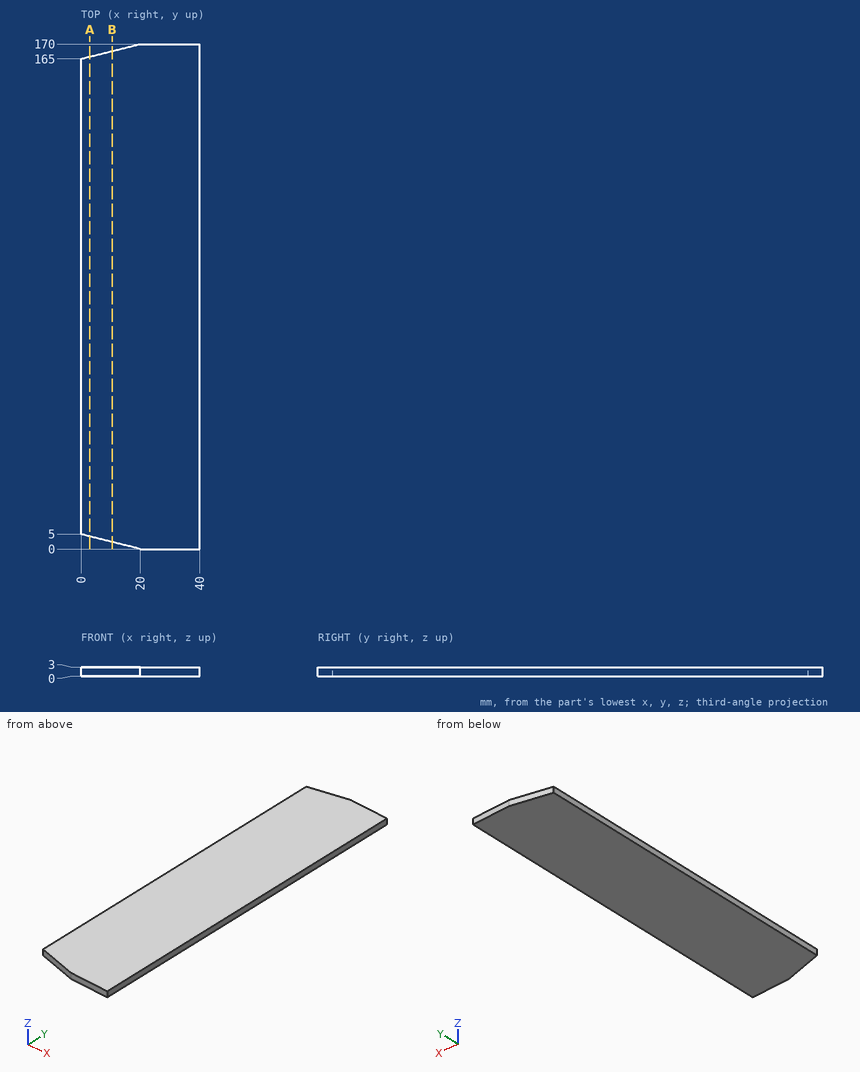
Geometry check sheet. Reference: drawing and pictorial views, mm from the part's lowest x, y, z. Round coordinates to 2 decimals unless told otherwise and drop trailing zeros. Loops run counter-clockwise (first coordinate to the right, second up) from the corner with the lowest first, then second, coordinate; pieces in that order, holes last. Notation, with made-up numbers: (62.25, -32.75) - (111.25, -32.75) arc R24 ccw to (111.25, -6.75) - close; hole circle Ø6 at (64.25, -37). An arc over 180 degrees is marked (long way). Answer in a Markdown table with one row per item. Add a question column.
Q1. Section check B-B on x = 10.5. Enter the section's corners in (y, z) (3 decimals), plus the area to 3 significant figures.
Q2. Material ranges on line 1 (Y direction, x = 10, z = 0.2); line 2 (Y direction, x = 12, z = 1.7), recorded low to high.
Q3. Section check A-A on x = 3. Enter the section's corners in (y, z).
Found:
| question | item | result |
|---|---|---|
| 1 | outline | (2.375, 0) - (167.625, 0) - (167.625, 3) - (2.375, 3) - close |
| 1 | area | 496 mm² |
| 2 | line 1 | y = 2.5 to 167.5 |
| 2 | line 2 | y = 2 to 168 |
| 3 | outline | (4.25, 0) - (165.75, 0) - (165.75, 3) - (4.25, 3) - close |
